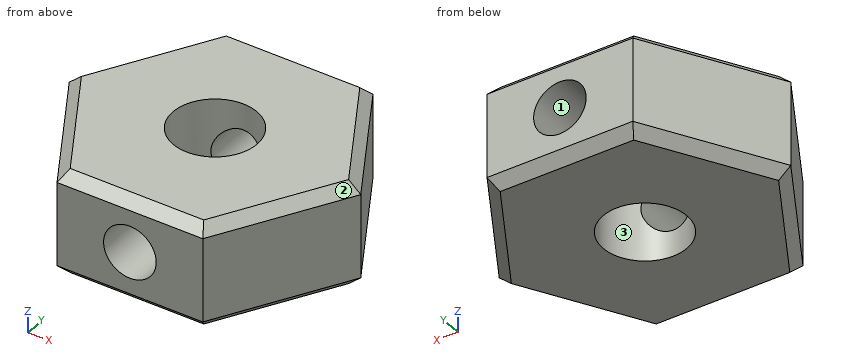
from build123d import *

# Parameters (mm, degrees)
SALIENTE_EXTRUIR1_DEPTH = 5
CROQUIS2_R              = 2
CORTAR_EXTRUIR1_DEPTH   = 5
CHAFL_N1_SIZE           = 0.5
CROQUIS3_R              = 1.25
CORTAR_EXTRUIR2_DEPTH   = 13


with BuildPart() as part:
    # Croquis1 → Saliente-Extruir1 (new body)
    with BuildSketch(Plane.XY):
        Polygon((6.92820323, 0), (3.464101615, 6), (-3.464101615, 6), (-6.92820323, 0), (-3.464101615, -6), (3.464101615, -6), align=None)
    extrude(amount=SALIENTE_EXTRUIR1_DEPTH)

    # Croquis2 → Cortar-Extruir1 (cut)
    with BuildSketch(Plane.XY.offset(5)):
        Circle(CROQUIS2_R)
    extrude(amount=-CORTAR_EXTRUIR1_DEPTH, mode=Mode.SUBTRACT)

    # Chaflán1
    chafl_n1_edges = [part.edges().sort_by_distance(p)[0] for p in [
        (0, 6, 5),
        (-5.196152423, 3, 5),
        (-5.196152423, -3, 5),
        (0, -6, 5),
        (5.196152423, -3, 5),
        (0, -6, 0),
        (-5.196152423, -3, 0),
        (-5.196152423, 3, 0),
        (5.196152423, 3, 5),
        (0, 6, 0),
        (5.196152423, 3, 0),
        (5.196152423, -3, 0),
    ]]
    chamfer(chafl_n1_edges, length=CHAFL_N1_SIZE)

    # Croquis3 → Cortar-Extruir2 (cut, through all)
    with BuildSketch(Plane(origin=(0, 6, 0), x_dir=(1, 0, 0), z_dir=(0, 1, 0))):
        with Locations((0, -2.5)):
            Circle(CROQUIS3_R)
    extrude(amount=-CORTAR_EXTRUIR2_DEPTH, mode=Mode.SUBTRACT)


solid = part.part
CAD build for the part. Positions are in the model's coordinates, mm. Face numbers are marked on the shaded views. Round coordinates to 2 decimals unless told otherwise and drop trailing zeros. Loops run counter-clockwise (first coordinate to the right, second up) from the corner with the lowest first, then second, coordinate; pieces in that order, holes last. Notation, with made-up numbers: M 25,-21.75 L 81,-21.75 A16 cw 81,-8.75 Z; hole C 30,9.25 d8. An arc over 180 degrees is marked long. One line per question, with ' | ' between items. Start each with the question number.
Item 1: Cut at A-A, the plane x = 0. Write the cut outline in (y, z), plus the area to 3 significant figures.
Item 2: Pin check, flat tips, straight feed: pin 1 Ø1 at (y, z) = (3, 2) entering from +X; pin 2 Ø2 at (x, z) = (0, 2.5) entering from +Y; pin 3 Ø2 at (y, z) = (4, 2.5) entering from +X. Stop position of each tip, or through.
Item 3: Wall check: line 1 (Z direction, x = 0, y = -4.1); line 2 (X direction, y = -1.5, z = 0.7); line 3 (X direction, y = 4.6, z = 2.5). Give the ranges that are in metal, low to high.
Item 4: Cut at C-C, the plane y = -2.5. Write the cut outline in (x, z).
Item 5: Cut at D-D, the plane x = -4.75. Write the cut outline in (y, z), plus the area to 3 significant figures.
Item 6: Cut at B-B, the plane z = 2.5. Write the cut outline in (x, y), plus the area to 3 significant figures.
Item 7: Two-plate mould, pull along Y, no slides. Class the marked faces 1, 2 and 3: pulls with the +Y half, pulls with the -Y half, needs draft (parallel to the pull), parting line crosses it, or undercut.
Responses:
1) outline: M -6,0.5 L -5.5,0 L -2,0 L -2,1.25 L -6,1.25 Z; M -6,3.75 L -2,3.75 L -2,5 L -5.5,5 L -6,4.5 Z; M 2,0 L 5.5,0 L 6,0.5 L 6,1.25 L 2,1.25 Z; M 2,3.75 L 6,3.75 L 6,4.5 L 5.5,5 L 2,5 Z | area: 19.5 mm²
2) pin 1: stops at x = 5.48 | pin 2: passes through | pin 3: stops at x = 5.2
3) line 1: z = 0 to 1.25, 3.75 to 5 | line 2: x = -6.06 to -1.32, 1.32 to 6.06 | line 3: x = -4.27 to -1.25, 1.25 to 4.27
4) outline: M -5.48,0.5 L -4.91,0 L 4.91,0 L 5.48,0.5 L 5.48,4.5 L 4.91,5 L -4.91,5 L -5.48,4.5 Z; hole C 0,2.5 d2.5
5) outline: M -3.77,0.5 L -2.77,0 L 2.77,0 L 3.77,0.5 L 3.77,4.5 L 2.77,5 L -2.77,5 L -3.77,4.5 Z | area: 36.7 mm²
6) outline: M -6.93,0 L -3.46,-6 L -1.25,-6 L -1.25,-1.56 A2 cw -1.25,1.56 L -1.25,6 L -3.46,6 Z; M 1.25,-6 L 3.46,-6 L 6.93,0 L 3.46,6 L 1.25,6 L 1.25,1.56 A2 cw 1.25,-1.56 Z | area: 91.4 mm²
7) face 1: needs draft | face 2: pulls with the -Y half | face 3: undercut
